```python
from build123d import *

# Parameters (mm, degrees)
F0_W     = 100
F0_H     = 900
F1_DEPTH = 20
F2_R     = 10
F3_DEPTH = 25


# Not quite as in the source:
# - a pattern or mirror of a feature is missing from the dataset's text; its kind, count and spacing are read off the source's solid


with BuildPart() as f1:
    # F0 (on Front) → F1 (new body)
    with BuildSketch(Plane.XZ):
        Rectangle(F0_W, F0_H)
    extrude(amount=F1_DEPTH)

    # F2 (on face) → F3 (cut)
    with BuildSketch(Plane.XZ.offset(20)):
        with Locations((0, -400)):
            Circle(F2_R)
    f3 = extrude(amount=-F3_DEPTH, mode=Mode.SUBTRACT)

    # F3_copies: F3 across plane
    add(f3.mirror(Plane.XY), mode=Mode.SUBTRACT)


solid = f1.part
```
Here's how the part is built. I have some questions about the finished solid (model axes, mm). Give positions to 0.01 mm unless a question says otherwise; leave off trailing zeros. Order: outer loops, then holes, each group sorted by start corner. A loop starts at its lowest first (then second) coordinate and runs counter-clockwise, first axis right, second up. Notation, with made-up numbers: (46, 64.25) -> (71, 64.25) arc R15 cw to (71, 74.25) -> close; hole circle Ø5 at (82, -27). An arc over 180 degrees is marked (long way). Use CSV: the item, a comma, the result in double quotes. Start each with the question number.
Item 1: Thinking about a two-plate mould opening in Z: for faces 1 (the flat face through (-1, -20, 6)), 2 (the cylindrical face through (-1.302, -10.14, -390.085)), 3 (the flat face through (-1, -10, 450)), which applies, pulls with the +Z half, pulls with the -Z half, needs draft (parallel to the pull), parting line crosses it, or undercut?
Item 2: If I drill on probe 1 along Z at (x, y) = (0, -13); probe 2 along X at (y, z) = (-6, 400); probe 3 along Z at (x, y) = (-7, -5.25), over which ranges is the centre line in solid material (lowest first)? Write a range as [from, to].
Item 3: Suppose I cut it at A-A (z = -400). List the corners of the cut face in (x, y) for me.
Item 4: Suppose I cut it at B-B (x = 0). List the corners of the cut face in (y, z) for me.
Answer block:
1,face 1,"needs draft"
1,face 2,"undercut"
1,face 3,"pulls with the +Z half"
2,probe 1,"z = [-450, -410], [-390, 390], [410, 450]"
2,probe 2,"x = [-50, -10], [10, 50]"
2,probe 3,"z = [-450, -407.14], [-392.86, 392.86], [407.14, 450]"
3,outline,"(-50, -20) -> (-10, -20) -> (-10, 0) -> (-50, 0) -> close; (10, -20) -> (50, -20) -> (50, 0) -> (10, 0) -> close"
4,outline,"(-20, -450) -> (0, -450) -> (0, -410) -> (-20, -410) -> close; (-20, -390) -> (0, -390) -> (0, 390) -> (-20, 390) -> close; (-20, 410) -> (0, 410) -> (0, 450) -> (-20, 450) -> close"
